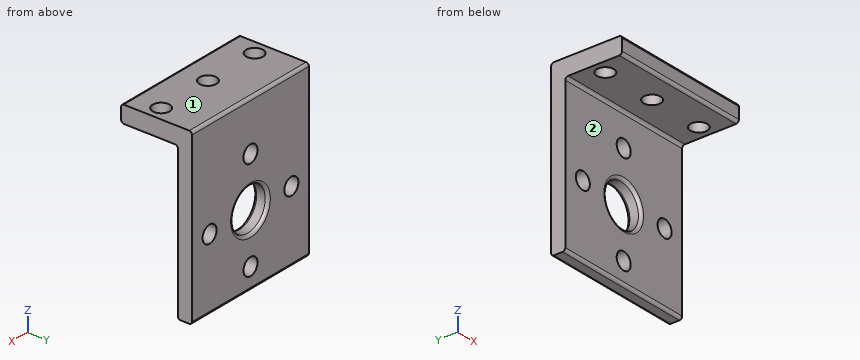
from build123d import *

# Parameters (mm, degrees)
SKETCH1_W           = 50
SKETCH1_H           = 50
SKETCH1_R           = 7.5
SKETCH1_R_2         = 3
BOSS_EXTRUDE1_DEPTH = 5
SKETCH2_W           = 50
SKETCH2_H           = 5
BOSS_EXTRUDE2_DEPTH = 10
SKETCH4_W           = 50
SKETCH4_H           = 6
BOSS_EXTRUDE3_DEPTH = 20
SKETCH5_R           = 3
CUT_EXTRUDE1_DEPTH  = 7
FILLET1_R           = 1


with BuildPart() as part:
    # Sketch1 → Boss-Extrude1 (new body)
    with BuildSketch(Plane(origin=(0, 0, 0), x_dir=(1, 0, 0), z_dir=(0, 1, 0))):
        Rectangle(SKETCH1_W, SKETCH1_H)
        Circle(SKETCH1_R, mode=Mode.SUBTRACT)
        with Locations((0, 17.5)):
            Circle(SKETCH1_R_2, mode=Mode.SUBTRACT)
        with Locations((17.5, 0)):
            Circle(SKETCH1_R_2, mode=Mode.SUBTRACT)
        with Locations((0, -17.5)):
            Circle(SKETCH1_R_2, mode=Mode.SUBTRACT)
        with Locations((-17.5, 0)):
            Circle(SKETCH1_R_2, mode=Mode.SUBTRACT)
    extrude(amount=BOSS_EXTRUDE1_DEPTH)

    # Sketch2 → Boss-Extrude2 (add)
    with BuildSketch(Plane.XY.offset(25)):
        with Locations((0, 2.5)):
            Rectangle(SKETCH2_W, SKETCH2_H)
    extrude(amount=BOSS_EXTRUDE2_DEPTH)

    # Sketch4 → Boss-Extrude3 (add)
    with BuildSketch(Plane.XZ):
        with Locations((0, 32)):
            Rectangle(SKETCH4_W, SKETCH4_H)
    extrude(amount=BOSS_EXTRUDE3_DEPTH)

    # Sketch5 → Cut-Extrude1 (cut, through all)
    with BuildSketch(Plane(origin=(0, 0, 29), x_dir=(-1, 0, 0), z_dir=(0, 0, -1))):
        with Locations((0, -10)):
            Circle(SKETCH5_R)
        with Locations((20, -10)):
            Circle(SKETCH5_R)
        with Locations((-20, -10)):
            Circle(SKETCH5_R)
    extrude(amount=-CUT_EXTRUDE1_DEPTH, mode=Mode.SUBTRACT)

    # Fillet1
    fillet1_edges = [part.edges().sort_by_distance(p)[0] for p in [
        (-7.5, 0, 0),
        (-7.5, 5, 0),
        (0, 5, 35),
        (0, 0, 29),
        (0, -20, 29),
        (0, -20, 35),
        (0, 0, -25),
        (0, 5, -25),
    ]]
    fillet(fillet1_edges, radius=FILLET1_R)


solid = part.part
The listing builds one solid part. Answer for the finished solid, in the listing's coordinates (mm). Face numbers are marked on the shaded views. A direction names the side the tool comes from. Round coordinates to 2 decimals unless told otherwise and drop trailing zeros. Write each loop counter-clockwise with the first axis right and the second up, starting at its lowest first coordinate (ties: lowest second). Pieces come first, ordered by that corner, then holes. Notation, with made-up numbers: (21.25, 79.25) - (63.25, 79.25) arc R28 ccw to (63.25, 115.25) - close; hole circle Ø3 at (-38.75, -21). An arc over 180 degrees is marked (long way). Use a Markdown table: item, result. Add a question column.
1. Flat-ended cylindrical pins translate along their axes: P1, Ø6, axis at x = -3, z = 0.5, coming from the -Y side; P2, Ø9.5, axis at x = -20, y = -10, coming from the -Z side; P3, Ø1, axis at x = -13, z = 28, coming from the -Y side; P4, Ø7, axis at x = 0, y = -10, coming from the +Z side. Find the tip coordinate at first contact, or state that the pin passes through.
2. The part is cut by section C-C (z = 0). Write down the section's boundary in (x, y).
3. A tool of negligible diameter and unlimited length cuts with its end or side. For the marked faces 1 and 2, from which of +Z, -Z, +X, -X, +Y, -Y can it reach the whole face along a straight path? Write none if from no direction.
4. Consider line 1 (X direction, y = 1.7, z = 0); line 2 (Z direction, x = -17.5, y = 3.7); line 3 (Z direction, x = -10.5, y = -7.5). Determine where each line is inside the solid, lowest interval first.
5. The part is cut by section B-B (y = -10). Write down the section's boundary in (x, z).
6. The part is cut by section A-A (z = -17.5). Write down the section's boundary in (x, y).
7. The part is cut by section D-D (x = -13). Write down the section's boundary in (y, z).
Reported:
| question | item | result |
|---|---|---|
| 1 | P1 | through |
| 1 | P2 | z = 29 |
| 1 | P3 | y = -0.13 |
| 1 | P4 | z = 35 |
| 2 | outline | (-25, 0) - (-20.5, 0) - (-20.5, 5) - (-25, 5) - close; (-14.5, 0) - (-8.5, 0) arc R1 ccw to (-7.5, 1) - (-7.5, 4) arc R1 ccw to (-8.5, 5) - (-14.5, 5) - close; (7.5, 1) arc R1 ccw to (8.5, 0) - (14.5, 0) - (14.5, 5) - (8.5, 5) arc R1 ccw to (7.5, 4) - close; (20.5, 0) - (25, 0) - (25, 5) - (20.5, 5) - close |
| 3 | face 1 | +Z, +X, -X, +Y, -Y |
| 3 | face 2 | -Z, +X, -X, -Y |
| 4 | line 1 | -25 to -20.5, -14.5 to -7.5, 7.5 to 14.5, 20.5 to 25 |
| 4 | line 2 | -25 to -3, 3 to 35 |
| 4 | line 3 | 29 to 35 |
| 5 | outline | (-25, 29) - (-23, 29) - (-23, 35) - (-25, 35) - close; (-17, 29) - (-3, 29) - (-3, 35) - (-17, 35) - close; (3, 29) - (17, 29) - (17, 35) - (3, 35) - close; (23, 29) - (25, 29) - (25, 35) - (23, 35) - close |
| 6 | outline | (-25, 0) - (-3, 0) - (-3, 5) - (-25, 5) - close; (3, 0) - (25, 0) - (25, 5) - (3, 5) - close |
| 7 | outline | (-20, 30) arc R1 ccw to (-19, 29) - (-1, 29) arc R1 cw to (0, 28) - (0, -24) arc R1 ccw to (1, -25) - (4, -25) arc R1 ccw to (5, -24) - (5, 34) arc R1 ccw to (4, 35) - (-19, 35) arc R1 ccw to (-20, 34) - close |
